from build123d import *

# Parameters (mm, degrees)
SKETCH_1_R          = 5
SKETCH_1_R_2        = 1.225
SKETCH_1_R_3        = 1.025
EXTRUDE_1_DEPTH     = 55
SKETCH_2_W          = 57.132931415
SKETCH_2_H          = 47
CUT_EXTRUDE_1_DEPTH = 66
SKETCH_3_R          = 1.25
CUT_EXTRUDE_2_DEPTH = 49
CUT_EXTRUDE_START   = -56
CUT_EXTRUDE_3_DEPTH = 56


with BuildPart() as part:
    # 스케치1 → 보스-돌출1 (new body)
    with BuildSketch(Plane.XY):
        with BuildLine():
            Line((11.674013781, 7.727703555), (-14, 46.512678751))
            Line((-14, 46.512678751), (-47.132931415, 46.512678751))
            Line((-47.132931415, 46.512678751), (-47.132931415, 14.921692086))
            Line((-47.132931415, 14.921692086), (-11, -8.660254038))
            ThreePointArc((-11, -8.660254038), (8.200906179, -11.346591463), (11.674013781, 7.727703555))
        make_face()
        Circle(SKETCH_1_R, mode=Mode.SUBTRACT)
        with Locations((0, 8)):
            Circle(SKETCH_1_R_2, mode=Mode.SUBTRACT)
        with Locations((0, 11)):
            Circle(SKETCH_1_R_2, mode=Mode.SUBTRACT)
        with Locations((7.778174593, 7.778174593)):
            Circle(SKETCH_1_R_2, mode=Mode.SUBTRACT)
        with Locations((8, 0)):
            Circle(SKETCH_1_R_2, mode=Mode.SUBTRACT)
        with Locations((11, 0)):
            Circle(SKETCH_1_R_2, mode=Mode.SUBTRACT)
        with Locations((7.778174593, -7.778174593)):
            Circle(SKETCH_1_R_2, mode=Mode.SUBTRACT)
        with Locations((0, -8)):
            Circle(SKETCH_1_R_2, mode=Mode.SUBTRACT)
        with Locations((0, -11)):
            Circle(SKETCH_1_R_2, mode=Mode.SUBTRACT)
        with Locations((-7.778174593, -7.778174593)):
            Circle(SKETCH_1_R_2, mode=Mode.SUBTRACT)
        with Locations((-8, 0)):
            Circle(SKETCH_1_R_3, mode=Mode.SUBTRACT)
        with Locations((-11, 0)):
            Circle(SKETCH_1_R_2, mode=Mode.SUBTRACT)
        with Locations((-7.778174593, 7.778174593)):
            Circle(SKETCH_1_R_2, mode=Mode.SUBTRACT)
    extrude(amount=EXTRUDE_1_DEPTH)

    # 스케치2 → 컷-돌출1 (cut)
    with BuildSketch(Plane(origin=(0, 46.512678751, 0), x_dir=(1, 0, 0), z_dir=(0, 1, 0))):
        with Locations((-14.566465708, -27.5)):
            Rectangle(SKETCH_2_W, SKETCH_2_H)
    extrude(amount=-CUT_EXTRUDE_1_DEPTH, mode=Mode.SUBTRACT)

    # 스케치3 → 컷-돌출2 (cut)
    with BuildSketch(Plane.ZY.offset(47.132931415)):
        with Locations(Location((24.5, 30.717185419, 0), (0, 0, 270))):
            Circle(SKETCH_3_R)
        with Locations(Location((14.5, 40.717185419, 0), (0, 0, 270))):
            Circle(SKETCH_3_R)
        with Locations(Location((34.5, 30.717185419, 0), (0, 0, 270))):
            Circle(SKETCH_3_R)
        with Locations(Location((24.5, 40.717185419, 0), (0, 0, 270))):
            Circle(SKETCH_3_R)
        with Locations(Location((14.5, 30.717185419, 0), (0, 0, 270))):
            Circle(SKETCH_3_R)
        with Locations(Location((34.5, 40.717185419, 0), (0, 0, 270))):
            Circle(SKETCH_3_R)
        with Locations(Location((14.5, 20.717185419, 0), (0, 0, 270))):
            Circle(SKETCH_3_R)
        with Locations(Location((24.5, 20.717185419, 0), (0, 0, 270))):
            Circle(SKETCH_3_R)
        with Locations(Location((34.5, 20.717185419, 0), (0, 0, 270))):
            Circle(SKETCH_3_R)
    extrude(amount=-CUT_EXTRUDE_2_DEPTH, mode=Mode.SUBTRACT)

    # 스케치4 → 컷-돌출3 (cut)
    with BuildSketch(Plane.XY.offset(55).offset(CUT_EXTRUDE_START)):
        with BuildLine():
            Line((-5, 0), (-5, -13.076696831))
            ThreePointArc((-5, -13.076696831), (0, -14), (5, -13.076696831))
            Line((5, -13.076696831), (5, 0))
            Line((5, 0), (-5, 0))
        make_face()
    extrude(amount=CUT_EXTRUDE_3_DEPTH, mode=Mode.SUBTRACT)


solid = part.part
Can you work these out from the model? Positions are in its coordinate system, mm. A direction names the side the tool comes from. Round coordinates to 2 decimals unless told otherwise and drop trailing zeros. Write each loop counter-clockwise with the first axis right and the second up, starting at its lowest first coordinate (ties: lowest second). Pieces come first, ordered by that corner, then holes. Notation, with made-up numbers: M -21.5,41 L 34.5,41 A17 cw 34.5,72 Z; hole C 4,15.5 d2. An arc over 180 degrees is marked long. Use CSV: the item, a comma, the result in double quotes.
(1) On a 3-axis mill with a long thin cutter (end or side, diameter ignored), from which of +Z, -Z, +X, -X, +Y, -Y can I reach the whole of each face in a straight line? I mean faces 1 (the cylindrical face through (8.343, -8.865, 1.972)), 2 (the flat face through (-43.133, 30, 28)), 3 (the flat face through (5, -7, 2)). Say none if no direction works.
Check values:
face 1,"+Z, -Z"
face 2,"+X, +Y, -Y"
face 3,"+Z, -Z, -Y"
(2) Imagine slicing it at A-A (z = 34.5). Write out the boundary of the cut face in (x, y).
Check values:
outline,"M -47.13,14.92 L -43.13,12.31 L -43.13,19.47 L -47.13,19.47 Z; M -47.13,21.97 L -43.13,21.97 L -43.13,29.47 L -47.13,29.47 Z; M -47.13,31.97 L -43.13,31.97 L -43.13,39.47 L -47.13,39.47 Z; M -47.13,41.97 L -43.13,41.97 L -43.13,46.51 L -47.13,46.51 Z"
(3) We'd pull the mould along Y, two halves only. Please class faces 4 (the cylindrical face through (-0.266, 6.804, 52.972)), 5 (the cylindrical face through (-8.342, -11.244, 1.972)), 6 (the cylindrical face through (13.276, -4.443, 1.972)), 7 (the cylindrical face through (6.776, 0.054, 1.972)): +Y half, -Y half, draft (parallel to the pull), parting line (faces both ways), or undercut.
Check values:
face 4,"undercut"
face 5,"-Y half"
face 6,"parting line"
face 7,"undercut"
(4) Imagine slicing it at D-D (y = 14). Write out the boundary of the cut face in (x, z).
Check values:
outline,"M -45.72,0 L 7.52,0 L 7.52,4 L -43.13,4 L -43.13,51 L 7.52,51 L 7.52,55 L -45.72,55 Z"
(5) Imagine slicing it at C-C (x = -36). Write out the boundary of the cut face in (y, z), plus the area to 3 significant figures.
Check values:
outline,"M 7.66,0 L 46.51,0 L 46.51,4 L 7.66,4 Z; M 7.66,51 L 46.51,51 L 46.51,55 L 7.66,55 Z"
area,"311 mm^2"
(6) I'm going to push flat-ended pins straight in: pin 1 (2 mm diameter, centred on y = 30.72, z = 34.5, fed in from -X); pin 2 (4 mm diameter, centred on y = 40.72, z = 34.5, fed in from +X); pin 3 (4.5 mm diameter, centred on y = -9.5, z = 2.5, fed in from -X). Where does each tip first touch, or does it pass through?
Check values:
pin 1,"through"
pin 2,"x = -43.13"
pin 3,"x = -13.16"
(7) I need wall thicknesses on line 1 along Z through (x, y) = (-10, 11); line 2 along Y through (x, z) = (-8, 1.75) (3 decimals); line 3 along X through (y, z) = (25.5, 47). Which ranges of each line are inside material? Lowest first, please.
Check values:
line 1,"0 to 4, 51 to 55"
line 2,"-11.489 to -8.983, -6.573 to -1.025, 1.025 to 6.573, 8.983 to 37.449"
line 3,"-47.13 to -43.13"
(8) Imagine slicing it at B-B (x = 0). Write out the boundary of the cut face in (y, z) (3 decimals), plus the area to 3 significant figures.
Check values:
outline,"M 5,0 L 6.775,0 L 6.775,4 L 5,4 Z; M 5,51 L 6.775,51 L 6.775,55 L 5,55 Z; M 9.225,0 L 9.775,0 L 9.775,4 L 9.225,4 Z; M 9.225,51 L 9.775,51 L 9.775,55 L 9.225,55 Z; M 12.225,0 L 25.363,0 L 25.363,4 L 12.225,4 Z; M 12.225,51 L 25.363,51 L 25.363,55 L 12.225,55 Z"
area,"124 mm^2"
